Design review of the part shown in the three views and the two pictorial views. Dimensions are in mm from the part's minimum x, y and z. A direction names the side the tool comes from. Give positions to 0.01 mm unless a question says otherwise; leave off trailing zeros. Order: outer loops, then holes, each group sorted by start corner. A loop starts at its lowest first (then second) coordinate and runs counter-clockwise, first axis right, second up. Notation, with made-up numbers: (-25, 29.5) -> (-10, 29.5) arc R14 cw to (-10, 35.5) -> close; hole circle Ø6 at (56, 80). An arc over 180 degrees is marked (long way). Use one line per item in the form item = value.
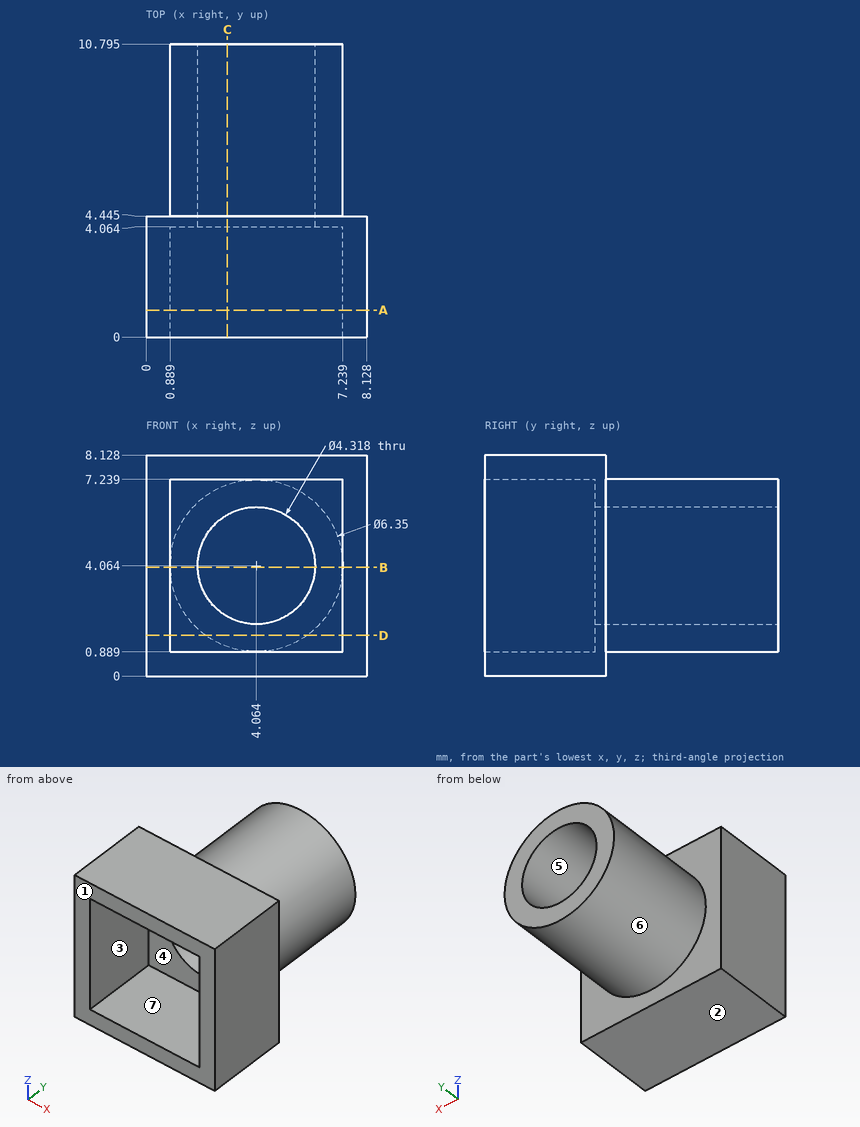
1. Add section D-D on z = 1.5. Give the boundary of the cut face in (x, y) (3 decimals), then the cut area to 3 significant figures.
Values:
outline = (0, 0) -> (0.889, 0) -> (0.889, 4.064) -> (7.239, 4.064) -> (7.239, 0) -> (8.128, 0) -> (8.128, 4.445) -> (5.937, 4.445) -> (5.937, 10.795) -> (2.191, 10.795) -> (2.191, 4.445) -> (0, 4.445) -> close
area = 34.1 mm^2
2. The part is to be moulded in two halves that separate along Z. For the marked faces 1, 2, 3 and 4, say which applies: +Z half, -Z half, draft (parallel to the pull), parting line (faces both ways), or undercut.
Values:
face_1 = draft
face_2 = -Z half
face_3 = undercut
face_4 = undercut
3. For L1, parallel to Z at x = 1.25, y = 1.25; L2, parallel to Z at x = 4, y = 9.75, list the stretches that pass through material, from the lowest coordinate up.
Values:
L1 = 0 to 0.89, 7.24 to 8.13
L2 = 0.89 to 1.91, 6.22 to 7.24
4. Tool access review of the marked faces 5, 6 and 7: name each direction out of +Z, -Z, +X, -X, +Y, -Y from which nothing blocks a thin tool from reaching the whole face with its end or side.
Values:
face_5 = +Y, -Y
face_6 = +Y
face_7 = -Y
5. Add section A-A on y = 1. Give the boundary of the cut face in (x, z).
Values:
outline = (0, 0) -> (8.13, 0) -> (8.13, 8.13) -> (0, 8.13) -> close; hole (0.89, 0.89) -> (7.24, 0.89) -> (7.24, 7.24) -> (0.89, 7.24) -> close
6. Add section C-C on x = 3. Give the boundary of the cut face in (y, z) (3 decimals), then the cut area to 3 significant figures.
Values:
outline = (0, 0) -> (4.445, 0) -> (4.445, 1.073) -> (10.795, 1.073) -> (10.795, 2.185) -> (4.064, 2.185) -> (4.064, 0.889) -> (0, 0.889) -> close; (0, 7.239) -> (4.064, 7.239) -> (4.064, 5.943) -> (10.795, 5.943) -> (10.795, 7.055) -> (4.445, 7.055) -> (4.445, 8.128) -> (0, 8.128) -> close
area = 23.0 mm^2
7. For pin 1 Ø1.5 at (y, z) = (7.5, 2.5) entering from -X; pin 2 Ø3 at (y, z) = (8, 6) entering from -X; pin 3 Ø1 at (x, y) = (5.5, 5) entering from -Z, all flat-tipped, find the tip position at first contact; note any pin that passes through.
Values:
pin_1 = 1
pin_2 = 0.92
pin_3 = 1.03
8. Add section B-B on z = 4. Give the boundary of the cut face in (x, y) (3 decimals).
Values:
outline = (0, 0) -> (0.889, 0) -> (0.889, 4.064) -> (1.906, 4.064) -> (1.906, 10.795) -> (0.89, 10.795) -> (0.89, 4.445) -> (0, 4.445) -> close; (6.222, 4.064) -> (7.239, 4.064) -> (7.239, 0) -> (8.128, 0) -> (8.128, 4.445) -> (7.238, 4.445) -> (7.238, 10.795) -> (6.222, 10.795) -> close
